Autodesk Inventor part; units mm, degrees
ref_plane "YZ Plane" through (0, 0, 0) normal (1, 0, 0) x (0, 1, 0)
ref_plane "XZ Plane" through (0, 0, 0) normal (0, 1, 0) x (-1, 0, 0)
ref_plane "XY Plane" through (0, 0, 0) normal (0, 0, 1) x (1, 0, 0)
sketch "Sketch2" plane through (0, 0, 0) normal (1, 0, 0) x (0, 1, 0)
  line L0 (127.2876, 96.9132) -> (-12.7124, 96.9132) construction
  line L1 (-12.7124, 96.9132) -> (-12.7124, -363.0868) construction
  line L2 (-12.7124, -363.0868) -> (127.2876, -363.0868) construction
  line L3 (127.2876, -363.0868) -> (127.2876, 96.9132) construction
  line L4 (97.2876, 66.9132) -> (17.2876, 66.9132) construction
  line L5 (17.2876, 66.9132) -> (17.2876, -333.0868) construction
  line L6 (17.2876, -333.0868) -> (97.2876, -333.0868) construction
  line L7 (97.2876, -333.0868) -> (97.2876, 66.9132) construction
  point P0 (0, 0)
  dimension "d2" = 140
  dimension "d3" = 460
  dimension "d4" = 80
  dimension "d5" = 400
  dimension "d6" = 30
  dimension "d7" = 30
sketch "Sketch3" plane through (0, 0, 0) normal (1, 0, 0) x (0, 1, 0)
  circle A0 centre (-62.7124, 66.9132) radius 20
  line L0 (-12.7124, 96.9132) -> (-12.7124, -363.0868) construction
  circle A1 centre (-62.7124, -13.0868) radius 20
  circle A2 centre (-62.7124, -93.0868) radius 20
  circle A3 centre (-62.7124, -173.0868) radius 20
  circle A4 centre (-62.7124, -253.0868) radius 20
  circle A5 centre (-62.7124, -333.0868) radius 20
  line L1 (127.2876, 96.9132) -> (-12.7124, 96.9132) construction
  point P0 (0, 0)
  dimension "d8" = 40
  dimension "d9" = 50
  dimension "d12" = 80
  dimension "d17" = 30
sketch "Sketch1" plane through (0, 0, 0) normal (1, 0, 0) x (0, 1, 0)
  circle A0 centre (45.5719, 146.9132) radius 40
  circle A1 centre (85.5719, -453.0868) radius 40
  line L0 (127.2876, 96.9132) -> (-12.7124, 96.9132) construction
  line L1 (-12.7124, -363.0868) -> (127.2876, -363.0868) construction
  line L2 (-62.7124, 66.9132) -> (-62.7124, -13.0868) construction
  line L3 (-62.7124, -253.0868) -> (-62.7124, -333.0868) construction
  line L4 (85.2399, 141.7706) -> (125.4799, -450.3748) construction
  circle A2 centre (-62.7124, 66.9132) radius 20
  line L5 (17.2876, 175.1975) -> (-76.8545, 81.0553)
  circle A3 centre (-62.7124, -333.0868) radius 20
  line L6 (-76.8545, -347.2289) -> (57.2876, -481.3711) construction
  point P0 (0, 0)
  dimension "d0" = 80
  dimension "d1" = 80
  dimension "d18" = 50
  dimension "d19" = 90
  dimension "d45" = 135
  dimension "d46" = 135
sketch "Sketch4" plane through (0, 0, 0) normal (1, 0, 0) x (0, 1, 0)
  line L0 (37.6815, -3.0868) -> (-57.7124, 26.9132) construction
  circle A0 centre (-62.7124, 66.9132) radius 20
  circle A1 centre (-62.7124, -13.0868) radius 20
  line L1 (-62.7124, 66.9132) -> (-62.7124, -13.0868) construction
  circle A2 centre (-27.7124, 112.5679) radius 20 construction
  circle A3 centre (-27.7124, 32.5679) radius 20 construction
  line L2 (-27.7124, 72.5679) -> (37.6815, -3.0868) construction
  line L3 (-27.7124, 72.5679) -> (-57.7124, 26.9132) construction
  line L4 (37.6815, -3.0868) -> (-42.7124, 49.7406) construction
  line L5 (-12.7124, 96.9132) -> (-12.7124, -363.0868) construction
  point P0 (0, 0)
  point P1 (-61.7124, 47.9132)
  point P2 (83.0715, 79.9132)
  point P3 (83.0715, -80.0868)
  point P4 (37.6815, -163.0868)
  point P5 (83.0715, -240.0868)
  point P6 (37.6815, -323.0868)
  dimension "d22" = 40
  dimension "d23" = 5
  dimension "d24" = 30
  dimension "d25" = 40
  dimension "d26" = 40
  dimension "d27" = 80
  dimension "d28" = 40
  dimension "d29" = 100
  dimension "d30" = 100
  dimension "d31" = 35
  dimension "d32" = 54.6292
  dimension "d33" = 27.3146
  dimension "d34" = 56.691
  dimension "d35" = 95.3939
  dimension "d36" = 45.39
  dimension "d37" = 83
  dimension "d40" = 160
sketch "Sketch6" plane through (0, 0, 0) normal (1, 0, 0) x (0, 1, 0)
  line L0 (234.6261, -208.0868) -> (-157.479, -208.0868) construction
  line L1 (237.7494, -58.0868) -> (-154.3557, -58.0868) construction
  line L2 (17.2876, -333.0868) -> (97.2876, -333.0868) construction
  line L3 (97.2876, 66.9132) -> (17.2876, 66.9132) construction
  point P0 (0, 0)
  dimension "d61" = 125
  dimension "d62" = 125
sketch "Sketch5" plane through (0, 0, 0) normal (1, 0, 0) x (0, 1, 0)
  arc A0 (90.5716, 146.9132) -> (47.894, 164.5909) centre (65.5716, 146.9132) ccw
  arc A1 (47.894, 164.5909) -> (90.5716, 146.9132) centre (65.5716, 146.9132) ccw construction
  line L0 (110.6559, 96.9132) -> (-29.3441, 96.9132) construction
  line L1 (-26.0812, -363.0868) -> (113.9188, -363.0868) construction
  line L2 (217.7491, -58.0868) -> (-174.356, -58.0868) construction
  line L3 (214.6258, -208.0868) -> (-177.4793, -208.0868) construction
  circle A2 centre (65.5716, 146.9132) radius 11
  circle A3 centre (65.5716, 146.9132) radius 55 construction
  line L4 (-10.2747, 106.4223) -> (47.894, 164.5909)
  line L5 (12.4387, 66.0715) -> (12.4387, -333.9285) construction
  line L6 (-62.7124, -14.3648) -> (-62.7124, -91.8088) construction
  line L7 (-62.7124, -173.0868) -> (-62.7124, -253.0868) construction
  line L8 (90.5716, -363.0868) -> (90.5716, -271.0908)
  line L9 (90.5716, -363.0868) -> (90.5716, -374.7257)
  arc A4 (82.3188, -382.1878) -> (90.5716, -374.7257) centre (83.0716, -374.7257) ccw
  arc A5 (11.0193, -373.8083) -> (14.9188, -375.3878) centre (15.6716, -367.9257) ccw
  line L10 (82.3188, -382.1878) -> (14.9188, -375.3878)
  arc A6 (-10.2747, -348.0868) -> (-3.3089, -362.4767) centre (8.0716, -348.0868) ccw
  line L11 (11.0193, -373.8083) -> (-3.3089, -362.4767)
  line L12 (-10.2747, -348.0868) -> (-10.2747, 106.4223)
  circle A7 centre (105.5716, -28.6718) radius 15 construction
  circle A8 centre (105.5716, -237.5018) radius 15 construction
  arc A9 (111.36, -33.441) -> (111.36, -23.9026) centre (105.5716, -28.6718) ccw
  arc A10 (111.36, -242.271) -> (111.36, -232.7326) centre (105.5716, -237.5018) ccw
  line L13 (111.36, -232.7326) -> (92.8538, -210.2717)
  line L14 (111.36, -242.271) -> (92.8538, -264.7319)
  line L15 (111.36, -33.441) -> (92.8538, -55.9019)
  line L16 (111.36, -23.9026) -> (92.8538, -1.4417)
  line L17 (90.5716, 4.9172) -> (90.5716, 146.9132)
  arc A11 (90.5716, 4.9172) -> (92.8538, -1.4417) centre (100.5716, 4.9172) ccw
  arc A12 (92.8538, -55.9019) -> (90.5716, -62.2608) centre (100.5716, -62.2608) ccw
  line L18 (90.5716, -203.9128) -> (90.5716, -62.2608)
  arc A13 (90.5716, -203.9128) -> (92.8538, -210.2717) centre (100.5716, -203.9128) ccw
  arc A14 (92.8538, -264.7319) -> (90.5716, -271.0908) centre (100.5716, -271.0908) ccw
  line L19 (127.2876, -363.0868) -> (127.2876, 96.9132) construction
  point P0 (0, 0)
  point P1 (83.0716, 81.9132)
  point P2 (83.0716, -348.0868)
  point P3 (16.3276, 122.4179)
  point P4 (8.0716, -82.4742)
  point P5 (8.0716, -243.0868)
  point P6 (-2.5613, -58.0868)
  point P7 (-2.5613, -208.0868)
  point P8 (8.0716, 81.9132)
  point P9 (-62.7124, 66.9132)
  point P10 (-62.7124, -333.0868)
  point P11 (-62.7124, -53.0868)
  point P12 (-62.7124, -213.0868)
  point P13 (2.2876, 6.9132)
  point P14 (45.3216, 26.9132)
  point P15 (50.3216, -93.0868)
  point P16 (7.2876, -113.0868)
  point P17 (7.2876, -153.0868)
  point P18 (50.3216, -173.0868)
  point P19 (45.3216, -293.0868)
  point P20 (2.2876, -273.0868)
  point P21 (2.2876, 6.9132)
  point P22 (-62.7124, 66.9132)
  point P23 (5.5716, -208.0868)
  point P24 (5.5716, -58.0868)
  point P25 (73.0216, -4.2568)
  point P26 (78.0216, -124.2568)
  point P27 (78.0216, -141.9168)
  point P28 (73.0216, -261.9168)
  point P29 (90.5716, -207.5018)
  point P30 (90.5716, -267.5018)
  point P31 (90.5716, -58.6718)
  point P32 (90.5716, 1.3282)
  point P33 (90.5716, -58.0868)
  point P34 (15.0521, -366.9249)
  dimension "d84" = 110
  dimension "d47" = 50
  dimension "d63" = 15
  dimension "d65" = 15
  dimension "d81" = 22
  dimension "d101" = 7.5
  dimension "d151" = 15
  dimension "d155" = 15
  dimension "d159" = 15
  dimension "d163" = 60
  dimension "d164" = 65
  dimension "d165" = 20
  dimension "d166" = 43.034
  dimension "d174" = 60
  dimension "d175" = 70
  dimension "d176" = 43.034
  dimension "d177" = 20
  dimension "d196" = 128.284
  dimension "d198" = 11.17
  dimension "d199" = 70.734
  dimension "d200" = 11.17
  dimension "d201" = 70.734
  dimension "d204" = 11.17
  dimension "d214" = 43.034
  dimension "d215" = 20
  dimension "d216" = 20
  dimension "d217" = 43.034
  dimension "d218" = 70.734
  dimension "d219" = 70.734
  dimension "d220" = 11.17
  dimension "d221" = 67.4
  dimension "d222" = 6.8
  dimension "d223" = 7.5
  dimension "d224" = 15
  dimension "d225" = 15
  dimension "d226" = 48.83
  dimension "d227" = 24.415
  dimension "d228" = 48.83
  dimension "d229" = 24.415
  dimension "d230" = 15
  dimension "d231" = 15
  dimension "d232" = 30
  dimension "d233" = 30
  dimension "d234" = 15
  dimension "d235" = 15
  dimension "d236" = 60
  dimension "d237" = 30
  dimension "d238" = 60
  dimension "d239" = 30
  dimension "d240" = 10
  dimension "d241" = 10
  dimension "d243" = 65
  dimension "d244" = 17.5
  dimension "d245" = 75
  dimension "d246" = 164.3874
extrude "Extrusion1" add sketch "Sketch5" against normal blind 5
hole "Hole1" at (0, 83.0716, 81.9132) at (0, 16.3276, 122.4179) at (0, 8.0716, -348.0868) at (0, 83.0716, -348.0868) at (0, -2.5613, -58.0868) at (0, -2.5613, -208.0868) at (0, 8.0716, 81.9132) at (0, 5.5716, -58.0868) at (0, 5.5716, -208.0868) at (0, 105.5716, -28.6718) at (0, 105.5716, -237.5018) direction (-1, 0, 0) diameter 5 end through all
hole "Otwór2" at (0, 2.2876, 6.9132) at (0, 45.3216, 26.9132) at (0, 7.2876, -113.0868) at (0, 50.3216, -93.0868) at (0, 7.2876, -153.0868) at (0, 50.3216, -173.0868) at (0, 2.2876, -273.0868) at (0, 45.3216, -293.0868) at (0, 83.0716, -374.7257) direction (-1, 0, 0) diameter 6 end through all
hole "Otwór3" at (0, 73.0216, -4.2568) at (0, 78.0216, -141.9168) at (0, 78.0216, -124.2568) at (0, 73.0216, -261.9168) at (0, 15.6716, -367.9257) direction (-1, 0, 0) diameter 5 end through all
equation "\"d28\" = 0.5 * d27"
equation "\"d30\" = d29"
equation "\"d33\" = 0.5 * d32"
equation "\"d62\" = d61"
properties part number "plyta_glowna_V3" material "Aluminium 6061"
Source: CAD feature listing. Evaluate the final solid. Frame: model axes, mm. A direction names the side the tool comes from. Give positions to 0.01 mm unless a question says otherwise; leave off trailing zeros. Loops run counter-clockwise (first coordinate to the right, second up) from the corner with the lowest first, then second, coordinate; pieces in that order, holes last. Notation, with made-up numbers: (-22, 88) - (0, 88) arc R23 ccw to (0, 96) - close; hole circle Ø4 at (-1, -35). An arc over 180 degrees is marked (long way). Use CSV: the item, a comma, the result in double quotes.
1) Set-up query: faces 1 (the flat face through (-2.465, 102.236, -221.659)), 2 (the cylindrical face through (-2.46, 75.52, 169.85)). Return all of +Z, -Z, +X, -X, +Y, -Y with unobstructed straight access to the full face (end or side cutting, diameter ignored); none if empty.
Worked out:
face 1,"+X, -X, +Y"
face 2,"+Z, +X, -X"
2) Cut plane A-A (y = 64.5). Output: boundary loops of the cut face in (x, z), and give its area (3 significant figures).
Worked out:
outline,"(-5, -380.39) - (0, -380.39) - (0, 135.97) - (-5, 135.97) - close; (-5, 157.86) - (0, 157.86) - (0, 171.89) - (-5, 171.89) - close"
area,"2,650 mm^2"
3) Line query: line 1 (Z direction, x = -3.2, y = 9.5); line 2 (Z direction, x = -0.2, y = 81); line 3 (Z direction, x = -2.8, y = 107.5). Output: solid intervals per line, ascending.
Worked out:
line 1,"z = -372.61 to -350.14, -346.04 to -155.11, -151.06 to -115.11, -111.06 to 79.86, 83.96 to 126.2"
line 2,"z = -382.05 to -376.9, -372.56 to -349.49, -346.69 to 80.51, 83.31 to 166.58"
line 3,"z = -246.96 to -239.09, -235.91 to -228.05, -38.13 to -30.26, -27.08 to -19.22"
4) Cut plane C-C (x = -3.35). Count the separate pieces of the cut face and the enclosed holes in it, and give its area (3 significant figures).
Worked out:
separate pieces,"1"
enclosed holes,"26"
area,"53,500 mm^2"
5) Pin query (flat end, axial travel): P1, Ø8, axis at y = 7.29, z = -153.09, coming from the -X side; P2, Ø2, axis at x = -1.5, y = 15, coming from the -Z side; P3, Ø1, axis at x = -1.5, z = -298, coming from the +Y side. Return the tip coordinate at first contact, or that it passes through.
Worked out:
P1,"stops at x = -5"
P2,"stops at z = -375.5"
P3,"stops at y = 90.57"
6) Cut plane B-B (z = 69.5). Output: boundary loops of the cut face in (x, y), and give its area (3 significant figures).
Worked out:
outline,"(-5, -10.27) - (0, -10.27) - (0, 90.57) - (-5, 90.57) - close"
area,"504 mm^2"
7) Cut plane D-D (y = 27.5). Output: boundary loops of the cut face in (x, z), and give its area (3 significant figures).
Worked out:
outline,"(-5, -376.66) - (0, -376.66) - (0, 144.2) - (-5, 144.2) - close"
area,"2,600 mm^2"
8) Mould query, pull axis Z, two halves, no side actions, for faces 3 (the flat face through (-5, 37, -101)), 4 (the flat face through (-2.465, 102.236, -12.829)), 5 (the cylindrical face through (-2.465, 54.582, 147.397)), 6 (the flat face through (-2.46, 102.24, -44.51)). Classes: +Z half, -Z half, draft (parallel to the pull), parting line (faces both ways), or undercut.
Worked out:
face 3,"draft"
face 4,"+Z half"
face 5,"undercut"
face 6,"undercut"
